Geometry: final body of the model. Coordinates: model frame, mm. A direction names the side the tool comes from. Round coordinates to 2 decimals unless told otherwise and drop trailing zeros. Loops run counter-clockwise (first coordinate to the right, second up) from the corner with the lowest first, then second, coordinate; pieces in that order, holes last. Notation, with made-up numbers: M 84.5,79 L 136.5,79 A7 cw 136.5,86 Z; hole C -16.75,-37 d8. An arc over 180 degrees is marked long. Answer as a JSON object with one key per item and string values.
from build123d import *

# Parameters (mm, degrees)
BOSS_EXTRUDE1_DEPTH = 5.15
SKETCH3_R           = 2.0675
CUT_EXTRUDE1_DEPTH  = 6.15


with BuildPart() as part:
    # Sketch1 → Boss-Extrude1 (new body)
    with BuildSketch(Plane.XY):
        Polygon((0, 0), (3, 0), (3, 8.97), (15, 8.97), (15, 0), (18, 0), (18, 20), (0, 20), align=None)
    extrude(amount=BOSS_EXTRUDE1_DEPTH)

    # Sketch3 → Cut-Extrude1 (cut, through all)
    with BuildSketch(Plane.XY.offset(5.15)):
        with Locations((9, 12.97)):
            Circle(SKETCH3_R)
    extrude(amount=-CUT_EXTRUDE1_DEPTH, mode=Mode.SUBTRACT)


solid = part.part
1) Pull-direction query (X, two-part tool) for faces 3 (the flat face through (3, 4, 3)), 4 (the flat face through (9, 20, 3)), 5 (the flat face through (0, 10, 3)); classes: +X half, -X half, draft (parallel to the pull), parting line (faces both ways), or undercut.
Results:
{"face 3": "undercut", "face 4": "draft", "face 5": "-X half"}
2) Pin query (flat end, axial travel): P1, Ø2.5, axis at y = 3, z = 2, coming from the -X side; P2, Ø2.5, axis at x = 9, y = 12.97, coming from the +Z side. Return the tip coordinate at first contact, or that it passes through.
Results:
{"P1": "x = 0", "P2": "through"}
3) Section query D-D (x = 13.25). Return the cut outline in (y, z).
Results:
{"outline": "M 8.97,0 L 20,0 L 20,5.15 L 8.97,5.15 Z"}
4) Section query A-A (y = 6.75). Return the cut outline in (x, z), and give its area (3 significant figures).
Results:
{"outline": "M 0,0 L 3,0 L 3,5.15 L 0,5.15 Z; M 15,0 L 18,0 L 18,5.15 L 15,5.15 Z", "area": "30.9 mm2"}
5) Section query C-C (x = 9). Return the cut outline in (y, z).
Results:
{"outline": "M 8.97,0 L 10.9,0 L 10.9,5.15 L 8.97,5.15 Z; M 15.04,0 L 20,0 L 20,5.15 L 15.04,5.15 Z"}
6) Section query B-B (z = 1.7). Return the cut outline in (x, y) (1 decimal).
Results:
{"outline": "M 0,0 L 3,0 L 3,9 L 15,9 L 15,0 L 18,0 L 18,20 L 0,20 Z; hole C 9,13 d4.1"}
7) Ray query, line 1 (X direction, y = 1.5, z = 1.85); line 2 (Y direction, x = 9, z = 3.65); line 3 (Y direction, x = 5.75, z = 3.75). Return the intervals inside material, ascending.
Results:
{"line 1": "0 to 3, 15 to 18", "line 2": "8.97 to 10.9, 15.04 to 20", "line 3": "8.97 to 20"}
8) Reachability of faces 1 (the flat face through (9, 8.97, 3)), 2 (the flat face through (7, 12, 0)) from +Z, -Z, +X, -X, +Y, -Y: full face, straight path, thin tool, end or side. Return the list, or none.
Results:
{"face 1": "+Z, -Z, -Y", "face 2": "-Z, +X, -X, +Y, -Y"}
